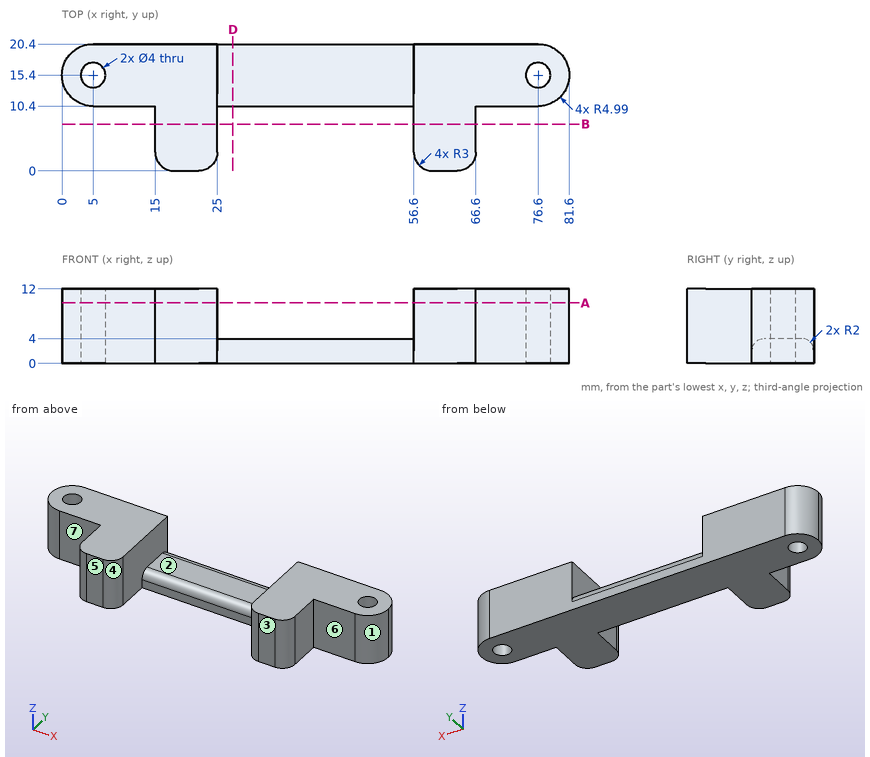
Check sheet for the drawn part. Datum: minimum x, y, z corner. Units: mm. A direction names the side the tool comes from. Coordinates: 2 decimals unless noted, no trailing zeros. Loops run counter-clockwise (first coordinate to the right, second up) from the corner with the lowest first, then second, coordinate; pieces in that order, holes last. Notation, with made-up numbers: (-10, 25) -> (-2, 25) arc R23 ccw to (-2, 63) -> close; hole circle Ø3 at (-33, 61). An arc over 180 degrees is marked (long way). Answer as a JSON object with one key per item and string values. Group by question number.
Item 1: Depth check by flat-ended pin: pin 1 (2 mm diameter, centred on y = 9, z = 7.5, fed in from +X); pin 2 (1.5 mm diameter, centred on y = 12.5, z = 6.5, fed in from +X); pin 3 (1.8 mm diameter, centred on x = 45.5, y = 14, fed in from +Z). Enter the tip coordinate at first touch or a pass-through.
Item 2: Sectioned sample at A-A on z = 9.75. State how many separate pieces and enclosed holes the cut face has, plus the area to 3 significant figures.
Item 3: Sectioned sample at D-D on x = 27.5. Record the boundary of the cut face in (y, z), plus the area to 3 significant figures.
Item 4: Tool access check on the marked faces 5, 6 and 7. Record the directions out of +Z, -Z, +X, -X, +Y, -Y that give a thin tool (end or side, any length) a straight path to the whole face; none if there is none.
Item 5: Scan lines: probe 1 along X at (y, z) = (8.5, 7.75); probe 2 along Y at (x, z) = (76.6, 7); probe 3 along Y at (x, z) = (31, 1). Record each from-to range of solid material in increasing order.
Item 6: Mould release check, pull along X, two halves, no side actions. Record for the marked faces 1, 2, 3 and 4: +X half, -X half, draft (parallel to the pull), parting line (faces both ways), or undercut.
Item 7: Sectioned sample at B-B on y = 7.5. Record the boundary of the cut face in (x, z).
Evaluation:
{
 "1": {"pin 1": "stops at x = 66.6", "pin 2": "stops at x = 81.12", "pin 3": "stops at z = 4"},
 "2": {"separate pieces": "2", "enclosed holes": "2", "area": "654 mm²"},
 "3": {"outline": "(10.4, 0) -> (20.4, 0) -> (20.4, 2) arc R2 ccw to (18.4, 4) -> (12.4, 4) arc R2 ccw to (10.4, 2) -> close", "area": "38.3 mm²"},
 "4": {"face 5": "+Z, -Z, +X, -X, -Y", "face 6": "+Z, -Z, +X, -Y", "face 7": "+Z, -Z, -X, -Y"},
 "5": {"probe 1": "x = 15 to 25, 56.6 to 66.6", "probe 2": "y = 10.4 to 13.4, 17.4 to 20.4", "probe 3": "y = 10.4 to 20.4"},
 "6": {"face 1": "+X half", "face 2": "undercut", "face 3": "draft", "face 4": "undercut"},
 "7": {"outline": "(15, 0) -> (25, 0) -> (25, 12) -> (15, 12) -> close; (56.6, 0) -> (66.6, 0) -> (66.6, 12) -> (56.6, 12) -> close"}
}
